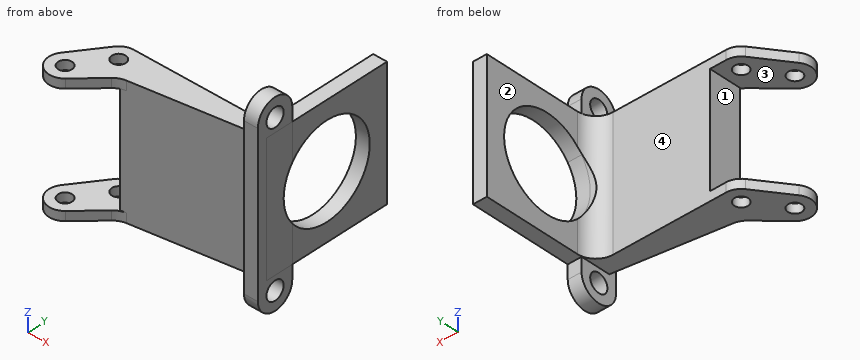
```python
from build123d import *

# Parameters (mm, degrees)
SKETCH2_R           = 3.5
SKETCH2_R_2         = 1.5
BOSS_EXTRUDE1_DEPTH = 2
BOSS_EXTRUDE2_START = -2
BOSS_EXTRUDE2_DEPTH = 2
BOSS_EXTRUDE3_START = -2
SKETCH4_R           = 1.5
BOSS_EXTRUDE3_DEPTH = 2
BOSS_EXTRUDE4_START = -26
SKETCH4_2_R         = 1.5
BOSS_EXTRUDE4_DEPTH = 2
BOSS_EXTRUDE5_START = -28
BOSS_EXTRUDE5_DEPTH = 28
FILLET1_R           = 4
CUT_EXTRUDE1_REACH  = 57.637
SKETCH6_R           = 10
SKETCH7_R           = 2
BOSS_EXTRUDE6_DEPTH = 3


with BuildPart() as part:
    # Sketch2 → Boss-Extrude1 (new body)
    with BuildSketch(Plane.XY):
        Circle(SKETCH2_R)
        Circle(SKETCH2_R_2, mode=Mode.SUBTRACT)
    extrude(amount=BOSS_EXTRUDE1_DEPTH)

    # Sketch3 → Boss-Extrude2 (add)
    with BuildSketch(Plane.XY.offset(2).offset(BOSS_EXTRUDE2_START)):
        with BuildLine():
            Line((3.5, 3.5), (0, 3.5))
            ThreePointArc((0, 3.5), (2.474873734, 2.474873734), (3.5, 0))
            Line((3.5, 0), (3.5, 3.5))
        make_face()
        with BuildLine():
            Line((3.5, -3.5), (3.5, 0))
            ThreePointArc((3.5, 0), (2.474873734, -2.474873734), (0, -3.5))
            Line((0, -3.5), (3.5, -3.5))
        make_face()
    extrude(amount=BOSS_EXTRUDE2_DEPTH)

    # Sketch4 → Boss-Extrude3 (add)
    with BuildSketch(Plane.XY.offset(2).offset(BOSS_EXTRUDE3_START)):
        with BuildLine():
            Line((-2.830776268, 2.058325952), (-7.920645724, -4.941674048))
            ThreePointArc((-7.920645724, -4.941674048), (-7.37878936, -9.647800157), (-2.64377537, -9.503322537))
            Line((-2.64377537, -9.503322537), (3.5, -3.5))
            Line((3.5, -3.5), (3.5, 3.5))
            Line((3.5, 3.5), (0, 3.5))
            ThreePointArc((0, 3.5), (-1.588373251, 3.118825166), (-2.830776268, 2.058325952))
        make_face()
        with Locations((-5.089869456, -7)):
            Circle(SKETCH4_R, mode=Mode.SUBTRACT)
        Circle(SKETCH4_R, mode=Mode.SUBTRACT)
    extrude(amount=BOSS_EXTRUDE3_DEPTH)



with BuildPart() as body_2:
    # Sketch4<2> → Boss-Extrude4 (new body)
    with BuildSketch(Plane.XY.offset(2).offset(BOSS_EXTRUDE4_START)):
        with BuildLine():
            Line((-2.830776268, 2.058325952), (-7.920645724, -4.941674048))
            ThreePointArc((-7.920645724, -4.941674048), (-7.37878936, -9.647800157), (-2.64377537, -9.503322537))
            Line((-2.64377537, -9.503322537), (3.5, -3.5))
            Line((3.5, -3.5), (3.5, 3.5))
            Line((3.5, 3.5), (0, 3.5))
            ThreePointArc((0, 3.5), (-1.588373251, 3.118825166), (-2.830776268, 2.058325952))
        make_face()
        with Locations((-5.089869456, -7)):
            Circle(SKETCH4_2_R, mode=Mode.SUBTRACT)
        Circle(SKETCH4_2_R, mode=Mode.SUBTRACT)
    extrude(amount=-BOSS_EXTRUDE4_DEPTH)


with BuildPart() as part_1:
    add(part.part)

    add(body_2.part)  # Boss-Extrude5 merges body 2
    # Sketch5 → Boss-Extrude5 (add)
    with BuildSketch(Plane.XY.offset(2).offset(BOSS_EXTRUDE5_START)):
        Polygon((3.5, 3.5), (28.5, 3.5), (28.5, 28.5), (31.5, 28.5), (31.5, 0.5), (3.5, -3.5), align=None)
    extrude(amount=BOSS_EXTRUDE5_DEPTH)

    # Fillet1
    fillet1_edges = [part_1.edges().sort_by_distance(p)[0] for p in [
        (3.5, -3.5, 1),
        (3.5, -3.5, -25),
        (28.5, 3.5, -12),
    ]]
    fillet(fillet1_edges, radius=FILLET1_R)

    # Sketch6 → Cut-Extrude1 (cut, up to next)
    with BuildSketch(Plane(origin=(31.5, 0, 0), x_dir=(0, 0, -1), z_dir=(1, 0, 0)), mode=Mode.PRIVATE) as cut_extrude1_sk1:
        with Locations((12, 14.5)):
            Circle(SKETCH6_R)
    cut_extrude1_tool1 = extrude(cut_extrude1_sk1.sketch, amount=-CUT_EXTRUDE1_REACH, mode=Mode.PRIVATE) & part_1.part
    add(cut_extrude1_tool1.solids().sort_by_distance((31.5, 14.5, -12))[0], mode=Mode.SUBTRACT)

    # Sketch7 → Boss-Extrude6 (add)
    # profile 1 of 2: a face of its own
    with BuildSketch(Plane(origin=(31.5, 0, 0), x_dir=(0, 0, -1), z_dir=(1, 0, 0))):
        with BuildLine():
            Line((6, 6.5), (-2, 6.5))
            Line((-2, 6.5), (-2, 0.5))
            Line((-2, 0.5), (26, 0.5))
            Line((26, 0.5), (26, 6.5))
            Line((26, 6.5), (18, 6.5))
            ThreePointArc((18, 6.5), (12, 4.5), (6, 6.5))
        make_face()
    # profile 2 of 2: a face of its own
    with BuildSketch(Plane(origin=(31.5, 0, 0), x_dir=(0, 0, -1), z_dir=(1, 0, 0))):
        with BuildLine():
            Line((-2, 6.5), (-5, 6.5))
            ThreePointArc((-5, 6.5), (-9, 2.5), (-5, -1.5))
            Line((-5, -1.5), (29, -1.5))
            ThreePointArc((29, -1.5), (33, 2.5), (29, 6.5))
            Line((29, 6.5), (26, 6.5))
            Line((26, 6.5), (26, 0.5))
            Line((26, 0.5), (-2, 0.5))
            Line((-2, 0.5), (-2, 6.5))
        make_face()
        with Locations((-5, 2.5)):
            Circle(SKETCH7_R, mode=Mode.SUBTRACT)
        with Locations((29, 2.5)):
            Circle(SKETCH7_R, mode=Mode.SUBTRACT)
    extrude(amount=-BOSS_EXTRUDE6_DEPTH)


solid = part_1.part
```
Read the model definition and answer for the solid it produces. Units are mm, in the model's axes. Face numbers are marked on the shaded views. A direction names the side the tool comes from. Give positions to 0.01 mm unless a question says otherwise; leave off trailing zeros. Write each loop counter-clockwise with the first axis right and the second up, starting at its lowest first coordinate (ties: lowest second). Pieces come first, ordered by that corner, then holes. Notation, with made-up numbers: (11, 13) - (25, 13) arc R14 cw to (25, 24) - close; hole circle Ø1 at (83, 36.5). An arc over 180 degrees is marked (long way). Write item = value, one per line. Start each with the question number.
Item 1: Find section D-D (y = 8.5). Give the vertices of the cut face in (x, z), then the cut area to 3 significant figures.
Item 2: A tool of negligible diameter and unlimited length cuts with its end or side. For the marked faces 1 and 2, from which of +Z, -Z, +X, -X, +Y, -Y can it reach the whole face along a straight path? Write none if from no direction.
Item 3: Find section B-B (z = -15). Give the vertices of the cut face in (x, y).
Item 4: Find the intervals of material crossed by probe 1 along Y at (x, z) = (29.5, -12); probe 2 along Z at (x, y) = (2.5, 2.5); probe 3 along Z at (x, y) = (14, 1), in increasing order. Write a range as [from, to].
Item 5: Find section A-A (y = 14.5). Give the vertices of the cut face in (x, z), then the cut area to 3 significant figures.
Item 6: The mould has two halves that part along Z. Classify the marked faces 3 and 4: +Z half, -Z half, draft (parallel to the pull), parting line (faces both ways), or undercut.
Item 7: Find section C-C (y = -7). Give the vertices of the cut face in (x, z), then the cut area to 3 significant figures.
Item 8: Each of these flat-tipped pins is pushed along its axis until it touches: P1, Ø2.5, axis at y = 2.5, z = -29, coming from the +X side; P2, Ø6, axis at y = 10, z = 4, coming from the -X side; P3, Ø0.9, axis at x = 30.5, z = -27.5, coming from the +Y side; P4, Ø2.5, axis at y = 2, z = -9, coming from the -X side. Where does it stop, or does it pass through?
Response:
q1.outline = (28.5, -26) - (31.5, -26) - (31.5, -20) - (28.5, -20) - close; (28.5, -4) - (31.5, -4) - (31.5, 2) - (28.5, 2) - close
q1.area = 36.0 mm²
q2.face_1 = -X, +Y, -Y
q2.face_2 = +Z, -Z, -X, +Y
q3.outline = (3.5, -3.5) - (28.5, 0.07) - (28.5, -1.5) - (31.5, -1.5) - (31.5, 4.96) - (27.59, 4.96) arc R4 cw to (24.5, 3.5) - (3.5, 3.5) - close; (28.5, 24.04) - (31.5, 24.04) - (31.5, 28.5) - (28.5, 28.5) - close
q4.probe_1 = [-1.5, 4.5], [24.5, 28.5]
q4.probe_2 = [-26, -24], [0, 2]
q4.probe_3 = [-26, 2]
q5.outline = (28.5, -26) - (31.5, -26) - (31.5, -22) - (28.5, -22) - close; (28.5, -2) - (31.5, -2) - (31.5, 2) - (28.5, 2) - close
q5.area = 24.0 mm²
q6.face_3 = undercut
q6.face_4 = draft
q7.outline = (-8.59, -26) - (-6.59, -26) - (-6.59, -24) - (-8.59, -24) - close; (-8.59, 0) - (-6.59, 0) - (-6.59, 2) - (-8.59, 2) - close; (-3.59, -26) - (-0.08, -26) - (-0.08, -24) - (-3.59, -24) - close; (-3.59, 0) - (-0.08, 0) - (-0.08, 2) - (-3.59, 2) - close
q7.area = 22.0 mm²
q8.P1 = through
q8.P2 = 28.5
q8.P3 = 6.5
q8.P4 = 3.5
